```python
from build123d import *

# Parameters (mm, degrees)
F1_DEPTH = 25.4
F2_R     = 5.08
F3_R     = 5.08
F4_SIZE  = 5.08


with BuildPart() as f1:
    # F0 (on Top) → F1 (new body)
    with BuildSketch(Plane.XY):
        with BuildLine():
            Line((-76.0381892323, -17.0626985246), (-76.0381892323, -37.1113419533))
            Line((-76.0381892323, -37.1113419533), (-53.9251491427, -37.1113419533))
            ThreePointArc((-53.9251491427, -37.1113419533), (-33.9361871958, -23.1446837303), (-26.2583127076, 0))
            ThreePointArc((-26.2583127076, 0), (-33.9361871958, 23.1446837303), (-53.9251491427, 37.1113419533))
            Line((-53.9251491427, 37.1113419533), (-76.0381892323, 37.1113419533))
            Line((-76.0381892323, 37.1113419533), (-76.0381892323, 17.0626985246))
            ThreePointArc((-76.0381892323, 17.0626985246), (-55.2712803961, 17.8631090788), (-44.6498636494, 0))
            ThreePointArc((-44.6498636494, 0), (-55.2712803961, -17.8631090788), (-76.0381892323, -17.0626985246))
        make_face()
        with BuildLine():
            ThreePointArc((-76.0381892323, 37.1113419533), (-103.7050256675, 0), (-76.0381892323, -37.1113419533))
            Line((-76.0381892323, -37.1113419533), (-76.0381892323, -17.0626985246))
            ThreePointArc((-76.0381892323, -17.0626985246), (-85.3134747257, 0), (-76.0381892323, 17.0626985246))
            Line((-76.0381892323, 17.0626985246), (-76.0381892323, 37.1113419533))
        make_face()
        with BuildLine():
            Line((-53.9251491427, -37.1113419533), (-76.0381892323, -37.1113419533))
            ThreePointArc((-76.0381892323, -37.1113419533), (-64.9816691875, -38.72335648), (-53.9251491427, -37.1113419533))
        make_face()
        with BuildLine():
            ThreePointArc((-26.2583127076, 0), (-33.9361871958, -23.1446837303), (-53.9251491427, -37.1113419533))
            Line((-53.9251491427, -37.1113419533), (76.0381892323, -37.1113419533))
            Line((76.0381892323, -37.1113419533), (76.0381892323, 37.1113419533))
            Line((76.0381892323, 37.1113419533), (-53.9251491427, 37.1113419533))
            ThreePointArc((-53.9251491427, 37.1113419533), (-33.9361871958, 23.1446837303), (-26.2583127076, 0))
        make_face()
        with BuildLine():
            ThreePointArc((-53.9251491427, 37.1113419533), (-64.9816691875, 38.72335648), (-76.0381892323, 37.1113419533))
            Line((-76.0381892323, 37.1113419533), (-53.9251491427, 37.1113419533))
        make_face()
    extrude(amount=F1_DEPTH)

    # F2
    f2_edges = [f1.edges().sort_by_distance(p)[0] for p in [
        (-85.313475, 0, 25.4),
    ]]
    fillet(f2_edges, radius=F2_R)

    # F3
    f3_edges = [f1.edges().sort_by_distance(p)[0] for p in [
        (-85.313475, 0, 0),
    ]]
    fillet(f3_edges, radius=F3_R)

    # F4
    f4_edges = [f1.edges().sort_by_distance(p)[0] for p in [
        (11.05652, -37.111342, 25.4),
        (11.05652, 37.111342, 25.4),
        (11.05652, -37.111342, 0),
    ]]
    chamfer(f4_edges, length=F4_SIZE)


solid = f1.part
```
Can you work these out from the model? Positions are in its coordinate system, mm. A direction names the side the tool comes from. Coordinates: 2 decimals unless noted, no trailing zeros. Loops run counter-clockwise (first coordinate to the right, second up) from the corner with the lowest first, then second, coordinate; pieces in that order, holes last.
Item 1: Suppose I cut it at A-A (z = 11.25). Please give me the cut outline in (x, y), then the cut area to 3 significant figures.
Answers below:
outline: (-53.93, -37.11) - (76.04, -37.11) - (76.04, 37.11) - (-53.93, 37.11) arc R38.72 ccw (long way) to start; hole circle Ø40.66 at (-64.98, 0)
area: 11,500 mm2
Item 2: Please list where these lines run through material, in increasing order: L1, parallel to Y at x = -66, z = 11.25; L2, parallel to X at y = -15, z = 19.25; L3, parallel to Y at x = -57, z = 17.5.
Answers below:
L1: y = -38.71 to -20.31, 20.31 to 38.71
L2: x = -100.68 to -78.71, -51.26 to 76.04
L3: y = -37.89 to -18.7, 18.7 to 37.89
Item 3: Which directions (+Z, -Z, +X, -X, +Y, -Y) give clear straight access to the entire face, cutting with the end or side of a thin tool? Please do faces 1 (the face through (10.15, -34.61, 2.58)), 2 (the face through (10, -37.111, 13)), 3 (the face through (11.97, 34.61, 22.82)), 4 (the face through (12, 37.111, 10)), 5 (the face through (10.15, -34.61, 22.82)).
Answers below:
face 1: -Z, +X, -Y
face 2: +Z, -Z, +X, -Y
face 3: +Z, +X, +Y
face 4: +Z, -Z, +X, +Y
face 5: +Z, +X, -Y
Item 4: Suppose I cut it at C-C (z = 1.75). Please give me the cut outline in (x, y).
Answers below:
outline: (-53.93, 37.11) arc R38.72 ccw (long way) to (-46.05, -33.78) - (76.04, -33.78) - (76.04, 37.11) - close; hole circle Ø43.15 at (-64.98, 0)
Item 5: Suppose I cut it at B-B (x = 26). Please give me the cut outline in (y, z).
Answers below:
outline: (-37.11, 5.08) - (-32.03, 0) - (37.11, 0) - (37.11, 20.32) - (32.03, 25.4) - (-32.03, 25.4) - (-37.11, 20.32) - close
Item 6: I'm going to push flat-ended pins straight in: pin 1 (10 mm diameter, centred on x = -53, z = 4, fed in from -Y); pin 2 (12 mm diameter, centred on x = 23, z = 11, fed in from -Y); pin 3 (3 mm diameter, centred on y = -30, z = 15.5, fed in from -X). Where does each tip first touch, or does it pass through?
Answers below:
pin 1: stops at y = -38.09
pin 2: stops at y = -37.11
pin 3: stops at x = -91.2
